Read the model definition and answer for the solid it produces. Units are mm, in the model's axes. Face numbers are marked on the shaded views. A direction names the side the tool comes from. Coordinates: 2 decimals unless noted, no trailing zeros. Loops run counter-clockwise (first coordinate to the right, second up) from the corner with the lowest first, then second, coordinate; pieces in that order, holes last.
from build123d import *

# Parameters (mm, degrees)
SKETCH1_R           = 6.35
BOSS_EXTRUDE1_DEPTH = 49.784
SKETCH2_W           = 33.02
SKETCH2_H           = 33.02
BOSS_EXTRUDE2_DEPTH = 5.842
SKETCH3_W           = 19.05
SKETCH3_H           = 26.67
BOSS_EXTRUDE3_DEPTH = 19.05


with BuildPart() as part:
    # Sketch1 → Boss-Extrude1 (new body)
    with BuildSketch(Plane(origin=(0, 0, 0), x_dir=(1, 0, 0), z_dir=(0, 1, 0))):
        with Locations(Location((0, 0, 0), (0, 0, 270))):
            Circle(SKETCH1_R)
    extrude(amount=BOSS_EXTRUDE1_DEPTH)

    # Sketch2 → Boss-Extrude2 (add)
    with BuildSketch(Plane.XZ):
        Rectangle(SKETCH2_W, SKETCH2_H)
    extrude(amount=BOSS_EXTRUDE2_DEPTH)

    # Sketch3 → Boss-Extrude3 (add)
    with BuildSketch(Plane.XZ.offset(5.842)):
        with Locations((0, -3.175)):
            Rectangle(SKETCH3_W, SKETCH3_H)
    extrude(amount=BOSS_EXTRUDE3_DEPTH)


solid = part.part
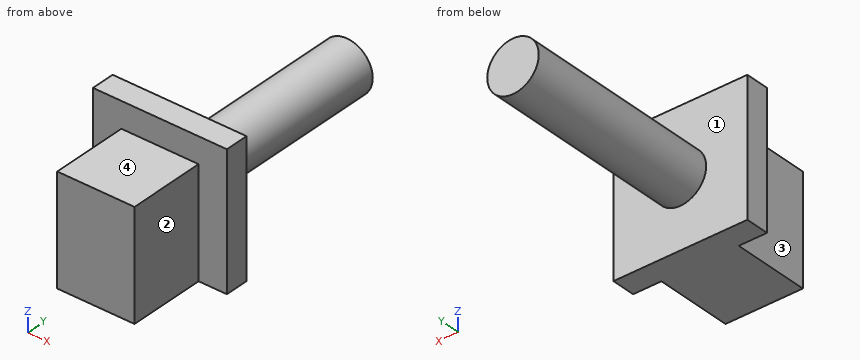
Q1. A cutting plane is placed at B-B (x = 0). Give the vertices of the cut face in (y, z), then the cut area to 3 significant figures.
Findings below:
outline: (-24.89, -16.51) - (0, -16.51) - (0, -6.35) - (49.78, -6.35) - (49.78, 6.35) - (0, 6.35) - (0, 16.51) - (-5.84, 16.51) - (-5.84, 10.16) - (-24.89, 10.16) - close
area: 1,330 mm2
Q2. Which of the six approach directions +Z, -Z, +X, -X, +Y, -Y give full straight-line access (tool end or side, diameter ignored) to the marked faces 1, 2, 3 and 4?
Findings below:
face 1: +Y
face 2: +Z, -Z, +X, -Y
face 3: +Z, -Z, -X, -Y
face 4: +Z, +X, -X, -Y
Q3. Straight lines are drawn through the part: probe 1 along Y at (x, z) = (5.5, -10); probe 2 along Z at (x, y) = (6, -21); probe 3 along X at (y, z) = (-11, -0.5) (3 decimals). For each, find the intervals that lie inside material, in ascending order.
Findings below:
probe 1: y = -24.89 to 0
probe 2: z = -16.51 to 10.16
probe 3: x = -9.525 to 9.525
Q4. A cutting plane is placed at D-D (z = 0). Give the vertices of the cut face in (x, y) (3 decimals).
Findings below:
outline: (-16.51, -5.842) - (-9.525, -5.842) - (-9.525, -24.892) - (9.525, -24.892) - (9.525, -5.842) - (16.51, -5.842) - (16.51, 0) - (6.35, 0) - (6.35, 49.784) - (-6.35, 49.784) - (-6.35, 0) - (-16.51, 0) - close
Q5. A cutting plane is placed at A-A (z = -10). Give the vertices of the cut face in (x, y) (3 decimals), then the cut area to 3 significant figures.
Findings below:
outline: (-16.51, -5.842) - (-9.525, -5.842) - (-9.525, -24.892) - (9.525, -24.892) - (9.525, -5.842) - (16.51, -5.842) - (16.51, 0) - (-16.51, 0) - close
area: 556 mm2
Q6. Flat-ended cylindrical pins translate along their axes: pin 1 Ø4 at (x, z) = (6, -9) entering from +Y; pin 2 Ø5.5 at (y, z) = (-14, -3) entering from +X (3 decimals); pin 3 Ø4 at (y, z) = (34.5, 0.5) entering from +X. Find the tip coordinate at first contact, or state that the pin passes through.
Findings below:
pin 1: stops at y = 0
pin 2: stops at x = 9.525
pin 3: stops at x = 6.35
Q7. A cutting plane is placed at C-C (y = 3). Give the vertices of the cut face in (x, z).
Findings below:
outline: circle Ø12.7 at (0, 0)
